CAD build for the part. Positions are in the model's coordinates, mm. Face numbers are marked on the shaded views. Round coordinates to 2 decimals unless told otherwise and drop trailing zeros. Write each loop counter-clockwise with the first axis right and the second up, starting at its lowest first coordinate (ties: lowest second). Pieces come first, ordered by that corner, then holes. Notation, with made-up numbers: (37, 8.25) - (43, 8.25) arc R22 cw to (43, 43.25) - close; hole circle Ø6 at (63.5, 44.5). An arc over 180 degrees is marked (long way). Answer in a Markdown table with one row per item.
```python
from build123d import *

# Parameters (mm, degrees)
SKETCH1_R           = 25
BOSS_EXTRUDE1_DEPTH = 364.692686
SKETCH2_R           = 19.544034105
CUT_EXTRUDE1_DEPTH  = 367.402449803


with BuildPart() as part:
    # Sketch1 → Boss-Extrude1 (new body)
    with BuildSketch(Plane(origin=(0, 0, 0), x_dir=(1, 0, 0), z_dir=(0, 1, 0))):
        with Locations(Location((0, 0, 0), (0, 0, 270))):
            Circle(SKETCH1_R)
    extrude(amount=BOSS_EXTRUDE1_DEPTH)

    # Sketch2 → Cut-Extrude1 (cut, through all)
    with BuildSketch(Plane(origin=(0, 0, 0), x_dir=(1, 0, 0), z_dir=(0, 1, 0))):
        with Locations(Location((0, 0, 0), (0, 0, 270))):
            Circle(SKETCH2_R)
    extrude(amount=CUT_EXTRUDE1_DEPTH, mode=Mode.SUBTRACT)

    # Chamfer1: read off the stored shape, not the designer's step
    # Chamfer1 outline → Chamfer1 (revolve, cut)
    with BuildSketch(Plane.XY):
        Polygon((25, 359.08197147), (25, 364.692686108), (19.544034105, 364.692686108), (19.544034105, 362.822599982), align=None)
        Polygon((25, 8.183616101), (19.544034105, 0.225711764), (19.544034105, 0), (25, 0), align=None)
    revolve(axis=Axis((0, 0, 0), (0, 1, 0)), mode=Mode.SUBTRACT)


solid = part.part
```
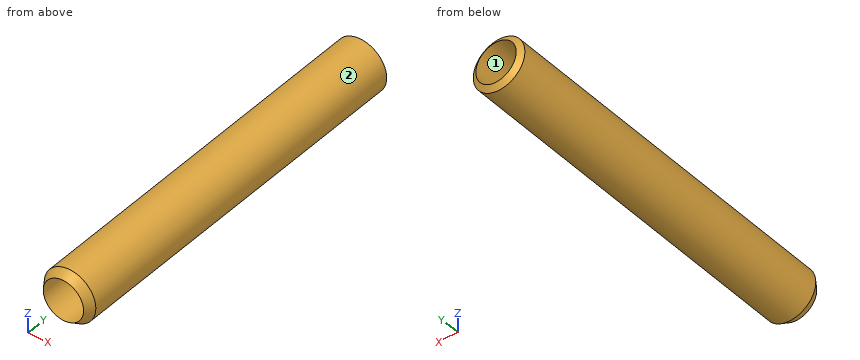
Q1. Drill centre lines: line 1 (X direction, y = 171, z = 0); line 2 (X direction, y = 289.5, z = -10.5); line 3 (Z direction, x = 2.5, y = 53.5). Where is each one in solid material? Low to high.
Computed:
| item | result |
|---|---|
| line 1 | x = -25 to -19.54, 19.54 to 25 |
| line 2 | x = -22.69 to -16.48, 16.48 to 22.69 |
| line 3 | z = -24.87 to -19.38, 19.38 to 24.87 |
Q2. Pull direction Z, two halves, no side cores. Call the marked faces 1 and 2: released by +Z, released by -Z, zero draft, split by the parting line, or undercut.
Computed:
| item | result |
|---|---|
| face 1 | undercut |
| face 2 | split by the parting line |
Q3. Saw through at C-C on y = 117.5. List the corners of the cut face in (x, z).
Computed:
| item | result |
|---|---|
| outline | circle Ø50 at (0, 0); hole circle Ø39.09 at (0, 0) |
Q4. Flat gauge pins, fed straight in: pin 1 (1 mm diameter, centred on y = 115, z = -10, fed in from -X); pin 2 (4 mm diameter, centred on x = -14, y = 130, fed in from -Z); pin 3 (4 mm diameter, centred on x = 15, y = 155, fed in from +Z); pin 4 (23.5 mm diameter, centred on x = 0, z = 0, fed in from +Y) (1 decimal). Where does each tip first touch, or does it go through?
Computed:
| item | result |
|---|---|
| pin 1 | stops at x = -23.12 |
| pin 2 | stops at z = -21.93 |
| pin 3 | stops at z = 21.35 |
| pin 4 | passes through |
Q5. Saw through at A-A on x = 0. List the corners of the cut face in (y, z), then the cut area to 3 significant figures.
Computed:
| item | result |
|---|---|
| outline | (0.23, -19.54) - (8.18, -25) - (359.08, -25) - (362.82, -19.54) - close; (0.23, 19.54) - (362.82, 19.54) - (359.08, 25) - (8.18, 25) - close |
| area | 3,890 mm2 |
Q6. Saw through at B-B on z = 0. List the corners of the cut face in (x, y).
Computed:
| item | result |
|---|---|
| outline | (-25, 8.18) - (-19.54, 0.23) - (-19.54, 362.82) - (-25, 359.08) - close; (19.54, 0.23) - (25, 8.18) - (25, 359.08) - (19.54, 362.82) - close |
